```python
from build123d import *

# Parameters (mm, degrees)
BOSS_EXTRUDE1_DEPTH = 100
FILLET1_R           = 1
SHELL3_T            = -0.2
SKETCH2_W           = 5.995745437
SKETCH2_H           = 2
CUT_EXTRUDE1_DEPTH  = 94


with BuildPart() as part:
    # Sketch1 → Boss-Extrude1 (new body)
    with BuildSketch(Plane(origin=(0, 0, 0), x_dir=(1, 0, 0), z_dir=(0, 1, 0))):
        Polygon((62.497660956, -33.372417048), (51.997660956, -31.04462309), (51.997660956, -36.54462309), (57.997660956, -36.54462309), (57.997660956, -40.54462309), (51.997660956, -40.54462309), (51.997660956, -46.04462309), (62.497660956, -43.716829132), align=None)
    extrude(amount=BOSS_EXTRUDE1_DEPTH)

    # Fillet1
    fillet1_edges = [part.edges().sort_by_distance(p)[0] for p in [
        (62.497660956, 50, 43.716829132),
        (51.997660956, 50, 46.04462309),
        (51.997660956, 50, 40.54462309),
        (57.997660956, 50, 40.54462309),
        (57.997660956, 50, 36.54462309),
        (51.997660956, 50, 36.54462309),
        (51.997660956, 50, 31.04462309),
        (62.497660956, 50, 33.372417048),
    ]]
    fillet(fillet1_edges, radius=FILLET1_R)

    # Shell3
    shell3_openings = [part.faces().sort_by_distance(p)[0] for p in [
        (57.425338322, 100, 32.431348777),
        (57.425338322, 0, 32.431348777),
    ]]
    offset(amount=SHELL3_T, openings=shell3_openings, kind=Kind.INTERSECTION)

    # Sketch2 → Cut-Extrude1 (cut)
    with BuildSketch(Plane(origin=(0, 100, 0), x_dir=(1, 0, 0), z_dir=(0, 1, 0))):
        with Locations((60.442884904, -38.54462309)):
            Rectangle(SKETCH2_W, SKETCH2_H)
    extrude(amount=-CUT_EXTRUDE1_DEPTH, mode=Mode.SUBTRACT)


solid = part.part
```
Read the model definition and answer for the solid it produces. Units are mm, in the model's axes. A direction names the side the tool comes from. Round coordinates to 2 decimals unless told otherwise and drop trailing zeros. Write each loop counter-clockwise with the first axis right and the second up, starting at its lowest first coordinate (ties: lowest second). Pieces come first, ordered by that corner, then holes. Notation, with made-up numbers: M 56.5,-18 L 82.5,-18 A16 cw 82.5,0 Z; hole C 48,-16.5 d1. An arc over 180 degrees is marked long. One line per item, written item: value.
Q1. Straight lines are drawn through the part: line 1 (X direction, y = 86, z = 34.5); line 2 (Z direction, x = 57, y = 33.5); line 3 (Z direction, x = 56.25, y = 19). For each, find the intervals that lie inside material, in ascending order. Write a range as [from, to].
Data:
line 1: [52, 52.2], [62.3, 62.5]
line 2: [32.15, 32.36], [36.34, 36.54], [40.54, 40.74], [44.73, 44.94]
line 3: [31.99, 32.19], [36.34, 36.54], [40.54, 40.74], [44.9, 45.1]
Q2. For a pull along X with two mould halves and no side action, classify faces 4 (the flat face through (51.998, 49, 34)), 5 (the flat face through (52.198, 49, 43)), 6 (the flat face through (55, 49, 40.545)), 7 (the flat face through (55, 49, 36.345)) as +X half, -X half, draft (parallel to the pull), parting line (faces both ways), or undercut.
Data:
face 4: -X half
face 5: undercut
face 6: draft
face 7: undercut
Q3. Find section B-B on x = 55. Write down the section's boundary in (y, z), plus the area to 3 significant figures.
Data:
outline: M 0,31.71 L 100,31.71 L 100,31.92 L 0,31.92 Z; M 0,36.34 L 100,36.34 L 100,36.54 L 0,36.54 Z; M 0,40.54 L 100,40.54 L 100,40.74 L 0,40.74 Z; M 0,45.17 L 100,45.17 L 100,45.38 L 0,45.38 Z
area: 81.0 mm2
Q4. Which of the six approach directions +Z, -Z, +X, -X, +Y, -Y give full straight-line access (tool end or side, diameter ignored) to faces 1 (the flat face through (58.198, 3, 39)), 2 (the flat face through (51.998, 49, 43)), 3 (the flat face through (57.998, 3, 39))?
Data:
face 1: +Y, -Y
face 2: +Z, -Z, -X, +Y, -Y
face 3: -X, +Y, -Y
Q5. Flat-ended cylindrical pins translate along their axes: pin 1 Ø6 at (x, y) = (53.5, 72) entering from -Z; pin 2 Ø1 at (y, z) = (3.5, 39) entering from -X; pin 3 Ø1 at (y, z) = (14, 39) entering from +X; pin 4 Ø2 at (x, y) = (59, 24.5) entering from +Z. Find the tip coordinate at first contact, or state that the pin passes through.
Data:
pin 1: z = 31.29
pin 2: x = 58
pin 3: through
pin 4: z = 44.71
Q6. Find section A-A on x = 60. Write down the section's boundary in (y, z), plus the area to 3 significant figures.
Data:
outline: M 0,32.82 L 100,32.82 L 100,33.02 L 0,33.02 Z; M 0,44.07 L 100,44.07 L 100,44.27 L 0,44.27 Z
area: 41.0 mm2
